The model under review builds one solid part; all positions refer to its coordinate system, in mm. A direction names the side the tool comes from. Coordinates: 2 decimals unless noted, no trailing zeros. Loops run counter-clockwise (first coordinate to the right, second up) from the corner with the lowest first, then second, coordinate; pieces in that order, holes last. Notation, with made-up numbers: M 13.25,84 L 55.25,84 A20 ccw 55.25,114 Z; hole C -3,-6.5 d7. An arc over 180 degrees is marked long. Write item = value, one per line. Start each with the question number.
Q1. For faces 1 (the face through (6, 240, -15)), 2 (the face through (21, 25, -6)), 3 (the face through (-4.309, -26.528, -7.327)), list the 3-axis set-ups (+Z, -Z, +X, -X, +Y, -Y) from which the entire face can be reached by the end or side of a thin tool; tool diameter is ignored.
Q2. Wall thickness on probe 1 along X at (y, z) = (-12.25, 0); probe 2 along Y at (x, z) = (-16.5, -19.5); probe 3 along X at (y, z) = (176, 15): over which ranges is each line inside the solid? List them lowest first.
Q3. Mouldability with a two-part tool opening along X and no side actions: class faces 4 (the face through (-21.317, 12.675, 2.799)), 5 (the face through (18.341, 36.042, 32.284)), 6 (the face through (0, 230, 22)) as released by +X, released by -X, zero draft, split by the parting line, or undercut.
Q4. We need section B-B on y = 45. Give the boundary of the cut face in (x, z), and give its area (3 significant figures).
Q5. Clearance check with flat-ended pins moving along their axes: pin 1 Ø5 at (x, z) = (14, -3) entering from +Y; pin 2 Ø5 at (x, z) = (0, 0) entering from -Y; pin 3 Ø1 at (x, y) = (14.5, 112) entering from -Z. State where each tip first meets the part, or that it passes through.
Q6. We need section A-A on y = 222.5. Give the boundary of the cut face in (x, z), and give its area (3 significant figures).
Q7. We need section C-C on y = 183. Give the boundary of the cut face in (x, z), and give its area (3 significant figures).
from build123d import *
from build123d.topology import SkipClean

# Parameters (mm, degrees)
SKIZZE2_W                       = 21.201346568
SKIZZE2_H                       = 40
AUFSATZ_LINEAR_AUSTRAGEN1_DEPTH = 41
SKIZZE3_R                       = 5.5
AUFSATZ_LINEAR_AUSTRAGEN2_DEPTH = 42
SKIZZE4_R                       = 4
SCHNITT_LINEAR_AUSTRAGEN1_DEPTH = 25
SKIZZE5_OUTSIDE_W               = 129.992
SKIZZE5_OUTSIDE_H               = 132.821
SCHNITT_LINEAR_AUSTRAGEN2_DEPTH = 4
SKIZZE6_W                       = 6
SKIZZE6_H                       = 22
AUFSATZ_LINEAR_AUSTRAGEN3_DEPTH = 37
VERRUNDUNG1_R                   = 4
AUFSATZ_LINEAR_START            = 20
AUFSATZ_LINEAR_AUSTRAGEN4_DEPTH = 20
SKIZZE8_W                       = 32
SKIZZE8_H                       = 16
SCHNITT_LINEAR_AUSTRAGEN3_DEPTH = 30
FASE1_SIZE                      = 18


with BuildPart() as part:
    # Skizze1 → Rotation1 (revolve)
    with BuildSketch(Plane.XY, mode=Mode.PRIVATE) as rotation1_sk:
        Polygon((8.5, 0), (21.5, 0), (21.5, 25), (25.75, 25), (33.75, 33), (33.75, 230), (0, 230), (0, -28.5), (11.5, -28.5), (11.5, -8), (8.5, -8), align=None)
    revolve(rotation1_sk.sketch.rotate(Axis((0, 0, 0), (0, 1, 0)), 90), axis=Axis((0, 0, 0), (0, 1, 0)))

    # Skizze2 → Aufsatz-Linear austragen1 (add)
    with BuildSketch(Plane.XY):
        with Locations((0, 80)):
            Rectangle(SKIZZE2_W, SKIZZE2_H)
    extrude(amount=AUFSATZ_LINEAR_AUSTRAGEN1_DEPTH)

    # Skizze3 → Aufsatz-Linear austragen2 (add)
    with BuildSketch(Plane.XZ.offset(-25)):
        with Locations(Location((33, 0, 0), (0, 0, 270))):
            Circle(SKIZZE3_R)
        with Locations(Location((-16.5, 28.578838325, 0), (0, 0, 270))):
            Circle(SKIZZE3_R)
        with Locations(Location((-16.5, -28.578838325, 0), (0, 0, 270))):
            Circle(SKIZZE3_R)
    extrude(amount=-AUFSATZ_LINEAR_AUSTRAGEN2_DEPTH)

    # Skizze4 → Schnitt-Linear austragen1 (cut)
    with BuildSketch(Plane.XZ.offset(28.5)):
        with Locations(Location((0, 0, 0), (0, 0, 270))):
            Circle(SKIZZE4_R)
    extrude(amount=-SCHNITT_LINEAR_AUSTRAGEN1_DEPTH, mode=Mode.SUBTRACT)

    # Skizze5 outside → Schnitt-Linear austragen2 (cut)
    with BuildSketch(Plane.XZ.offset(28.5)):
        with Locations((2.375, 3.4605)):
            Rectangle(SKIZZE5_OUTSIDE_W, SKIZZE5_OUTSIDE_H)
        Polygon((-8.5, -4.907477288), (0, -9.814954576), (8.5, -4.907477288), (8.5, 4.907477288), (0, 9.814954576), (-8.5, 4.907477288), align=None, mode=Mode.SUBTRACT)
    extrude(amount=-SCHNITT_LINEAR_AUSTRAGEN2_DEPTH, mode=Mode.SUBTRACT)

    # Skizze6 → Aufsatz-Linear austragen3 (add)
    with BuildSketch(Plane(origin=(0, 0, 0), x_dir=(0, 1, 0), z_dir=(0.7071067811865488, 0, 0.7071067811865464))):
        with Locations((36, 0)):
            Rectangle(SKIZZE6_W, SKIZZE6_H)
    extrude(amount=AUFSATZ_LINEAR_AUSTRAGEN3_DEPTH)

    # Verrundung1
    verrundung1_edges = [part.edges().sort_by_distance(p)[0] for p in [
        (18.384776311, 36, 33.941125497),
        (33.941125497, 36, 18.384776311),
    ]]
    fillet(verrundung1_edges, radius=VERRUNDUNG1_R)

    # Skizze7 → Aufsatz-Linear austragen4 (add)
    with SkipClean():  # the faces are left unmerged after this step: merging them gives an invalid solid
        with BuildSketch(Plane(origin=(0, 230, 0), x_dir=(1, 0, 0), z_dir=(0, 1, 0)).offset(AUFSATZ_LINEAR_START)):
            with BuildLine():
                Line((-30.233466556, 15), (30.233466556, 15))
                ThreePointArc((30.233466556, 15), (33.75, 0), (30.233466556, -15))
                Line((30.233466556, -15), (-30.233466556, -15))
                ThreePointArc((-30.233466556, -15), (-33.75, 0), (-30.233466556, 15))
            make_face()
        extrude(amount=-AUFSATZ_LINEAR_AUSTRAGEN4_DEPTH)

    # Skizze8 → Schnitt-Linear austragen3 (cut)
    with SkipClean():  # the faces are left unmerged after this step: merging them gives an invalid solid
        with BuildSketch(Plane(origin=(0, 250, 0), x_dir=(1, 0, 0), z_dir=(0, 1, 0))):
            with Locations((12, 0)):
                Rectangle(SKIZZE8_W, SKIZZE8_H)
        extrude(amount=-SCHNITT_LINEAR_AUSTRAGEN3_DEPTH, mode=Mode.SUBTRACT)

    # Fase1
    fase1_edges = [part.edges().sort_by_distance(p)[0] for p in [
        (-33.75, 250, 0),
    ]]
    chamfer(fase1_edges, length=FASE1_SIZE)


solid = part.part
Returned:
q1.face_1 = -Z, +X, -X, +Y
q1.face_2 = -Y
q1.face_3 = -Z, -X, -Y
q2.probe_1 = -11.5 to -4, 4 to 11.5
q2.probe_2 = 25 to 230
q2.probe_3 = -30.23 to 30.23
q3.face_4 = split by the parting line
q3.face_5 = undercut
q3.face_6 = zero draft
q4.outline = M -21.41,-26.09 A5.5 ccw -11.89,-31.58 A33.75 ccw 33.3,-5.49 A5.5 ccw 33.3,5.49 A33.75 ccw -11.89,31.58 A5.5 ccw -21.41,26.09 A33.75 ccw Z
q4.area = 3,700 mm^2
q5.pin_1 = 220
q5.pin_2 = -3.5
q5.pin_3 = -30.71
q6.outline = C 0,0 d67.5; hole M -4,-8 L 28,-8 L 28,8 L -4,8 Z
q6.area = 3,070 mm^2
q7.outline = C 0,0 d67.5
q7.area = 3,580 mm^2
